Input: part model. Units: mm. Frame: model coordinates. A direction names the side the tool comes from. Coordinates: 2 decimals unless noted, no trailing zeros. Order: outer loops, then holes, each group sorted by start corner. A loop starts at its lowest first (then second) coordinate and runs counter-clockwise, first axis right, second up. Notation, with made-up numbers: M 82.5,-4 L 118.5,-4 A21 cw 118.5,17 Z; hole C 56,0 d1. An arc over 180 degrees is marked long. One line per item, written item: value.
```python
from build123d import *

# Parameters (mm, degrees)
F1_R     = 40
F2_DEPTH = 25
F4_DEPTH = 3
F5_R     = 2


with BuildPart() as f2:
    # F1 (on face) → F2 (new body)
    with BuildSketch(Plane.XY):
        Circle(F1_R)
    extrude(amount=F2_DEPTH)

    # F3 (on face) → F4 (join)
    with BuildSketch(Plane.XY):
        with BuildLine():
            Line((-40.620192, -12.5), (40.620192, -12.5))
            ThreePointArc((40.620192, -12.5), (42.5, 0), (40.620192, 12.5))
            Line((40.620192, 12.5), (-40.620192, 12.5))
            ThreePointArc((-40.620192, 12.5), (-42.5, 0), (-40.620192, -12.5))
        make_face()
    extrude(amount=F4_DEPTH)

    # F5
    f5_edges = [f2.edges().sort_by_distance(p)[0] for p in [
        (-40, 0, 25),
    ]]
    fillet(f5_edges, radius=F5_R)


solid = f2.part
```
(1) Ray query, line 1 (Y direction, x = 0.5, z = 8.5); line 2 (Y direction, x = 37, z = 5); line 3 (X direction, y = 7.5, z = 19.25). Return the intervals inside material, ascending. Write a range as from..to.
Data:
line 1: y = -40..40
line 2: y = -15.2..15.2
line 3: x = -39.29..39.29
(2) Access query for faces 1 (the flat face through (-41, 0, 3)), 2 (the flat face through (39, 12.5, 1)), 3 (the flat face through (-39, -12.5, 1)), 4 (the flat face through (39, -12.5, 1)). Directions: +Z, -Z, +X, -X, +Y, -Y. A direction counts if a zero-diameter tool reaches every point of the face in a straight line with its end or side. Return the directions, or none.
Data:
face 1: +Z, -X
face 2: +Z, -Z, +X, +Y
face 3: +Z, -Z, -X, -Y
face 4: +Z, -Z, +X, -Y
(3) Cut plane B-B on z = 11.25. Output: boundary loops of the cut face in (x, y), plus the area to 3 significant figures.
Data:
outline: C 0,0 d80
area: 5,030 mm2
(4) Cut plane A-A on y = 0. Output: boundary loops of the cut face in (x, z), plus the area to 3 significant figures.
Data:
outline: M -42.5,0 L 42.5,0 L 42.5,3 L 40,3 L 40,23 A2 ccw 38,25 L -38,25 A2 ccw -40,23 L -40,3 L -42.5,3 Z
area: 2,010 mm2
(5) First-contact query: pin 1 (1.3 mm diameter, centred on x = -39, z = 2, fed in from +Y); pin 2 (1.5 mm diameter, centred on x = -14, z = 19.5, fed in from -Y); pin 3 (3.5 mm diameter, centred on x = -40.5, y = 3.5, fed in from +Z). Flat tips, straight axial feed; report the tip coordinate or a pass-through.
Data:
pin 1: stops at y = 12.5
pin 2: stops at y = -37.74
pin 3: stops at z = 24.79
